Check sheet for the drawn part. Datum: minimum x, y, z corner. Units: mm. Coordinates: 2 decimals unless noted, no trailing zeros. Write each loop counter-clockwise with the first axis right and the second up, starting at its lowest first coordinate (ties: lowest second). Pieces come first, ordered by that corner, then holes. Notation, with made-up numbers: (31, -16.75) - (83, -16.75) arc R22 cw to (83, 5.25) - close; hole circle Ø2 at (85, -13). An arc over 180 degrees is marked (long way). Use one line per item in the form item = value. Start each with the question number.
1. Cross-section at A-A on z = 5.95. Record the boundary of the cut face in (x, y).
2. Go/stop test with flat-tipped pins: pin 1 Ø2 at (y, z) = (12.5, 8.5) entering from +X; pin 2 Ø1.8 at (x, z) = (5.95, 5.95) entering from +Y; pin 3 Ø3.5 at (x, z) = (4, 3.5) entering from -Y. Record where each tip stops, or that it passes through.
3. Scan lines: line 1 along X through (y, z) = (12.3, 5.95); line 2 along Y through (x, z) = (8, 3.75); line 3 along Z through (x, y) = (8.75, 8.5). Record each from-to range of solid material in increasing order.
4. Cross-section at B-B on y = 4.25. Record the boundary of the cut face in (x, z).
5. Draft check along Z on the marked faces 1, 2 and 3. Enter one of: +Z half, -Z half, draft (parallel to the pull), parting line (faces both ways), or undercut.
6. Cross-section at C-C on x = 5.95. Record the boundary of the cut face in (y, z), then the cut area to 3 significant figures.
7. Cross-section at D-D on y = 7.5. Record the boundary of the cut face in (x, z).
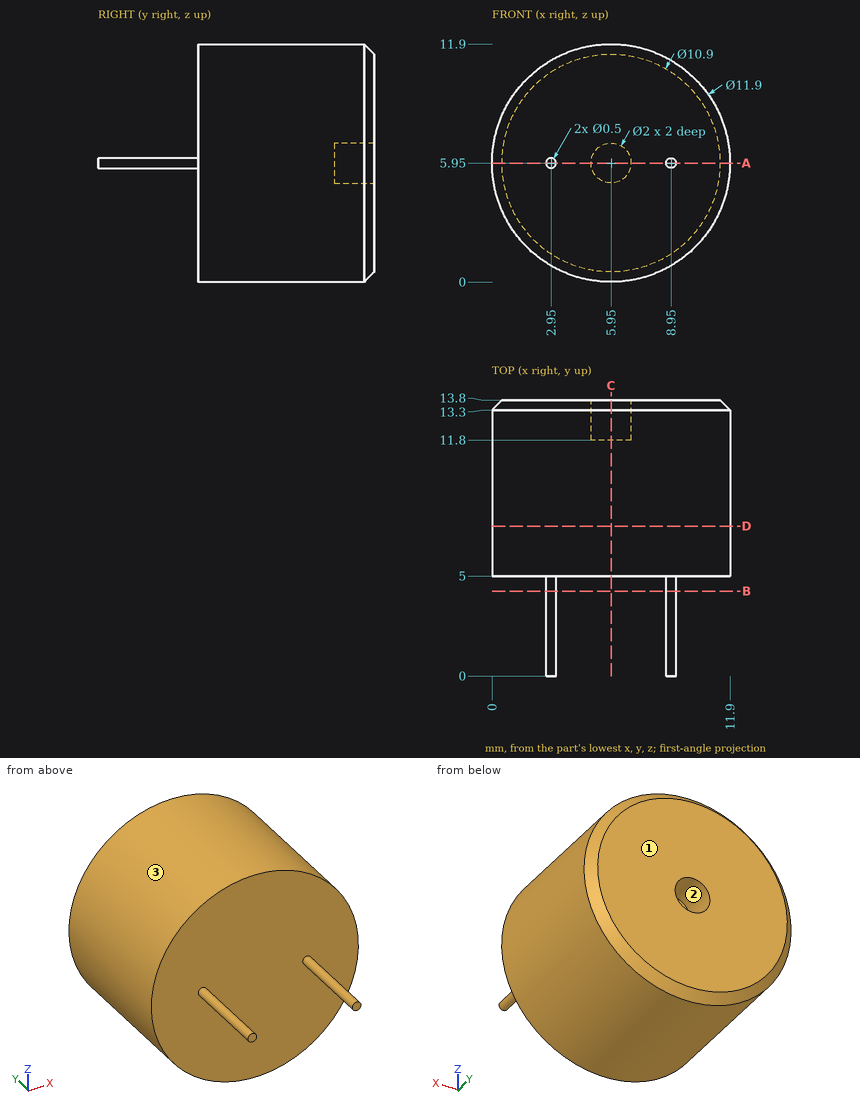
Final values:
q1.outline = (0, 5) - (2.7, 5) - (2.7, 0) - (3.2, 0) - (3.2, 5) - (8.7, 5) - (8.7, 0) - (9.2, 0) - (9.2, 5) - (11.9, 5) - (11.9, 13.3) - (11.4, 13.8) - (6.95, 13.8) - (6.95, 11.8) - (4.95, 11.8) - (4.95, 13.8) - (0.5, 13.8) - (0, 13.3) - close
q2.pin_1 = 11.69
q2.pin_2 = 11.8
q2.pin_3 = 5
q3.line_1 = 0 to 4.95, 6.95 to 11.9
q3.line_2 = 5 to 13.8
q3.line_3 = 0.7 to 11.2
q4.outline = circle Ø0.5 at (2.95, 5.95); circle Ø0.5 at (8.95, 5.95)
q5.face_1 = draft
q5.face_2 = undercut
q5.face_3 = parting line
q6.outline = (5, 0) - (13.3, 0) - (13.8, 0.5) - (13.8, 4.95) - (11.8, 4.95) - (11.8, 6.95) - (13.8, 6.95) - (13.8, 11.4) - (13.3, 11.9) - (5, 11.9) - close
q6.area = 100 mm²
q7.outline = circle Ø11.9 at (5.95, 5.95)
